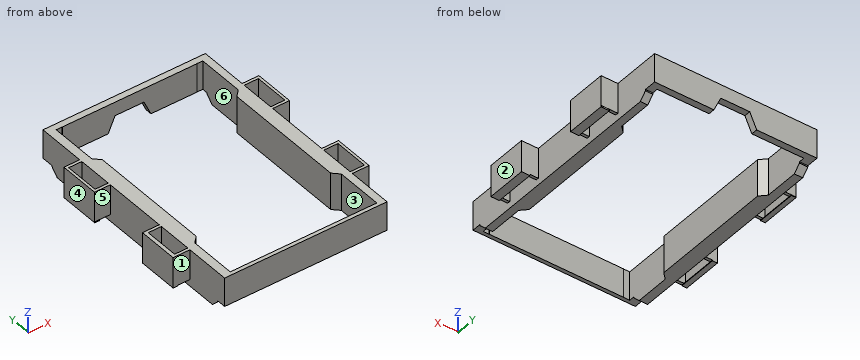
```python
from build123d import *

# Parameters (mm, degrees)
F0_W          = 60.96
F0_H          = 91.44
F0_W_2        = 50.8
F0_H_2        = 86.614
F1_DEPTH      = 28.448
F3_DEPTH      = 25.4
F4_W          = 66.649839282
F4_H          = 6.9823637605
F5_DEPTH      = 3.048
F6_W          = 64.9686481762
F6_H          = 4.777956934
F7_DEPTH      = 3.048
F9_DEPTH      = 2.286
F10_W         = 99.848318845
F10_H         = 48.2080141082
F11_DEPTH     = 50.8
F13_T1_DEPTH  = 15.8581495789
F13_T3_DEPTH  = 15.8581495789
F13_T8_DEPTH  = 41.5121495789
F13_T13_DEPTH = 41.5121495789
F13_T18_DEPTH = 41.5121495789
F13_T23_DEPTH = 41.5121495789
F14_W         = 15.24
F14_H         = 23.368
F15_DEPTH     = 6.35
F16_W         = 5.3607832682
F16_H         = 13.1506472826
F17_DEPTH     = 25.909
F19_DEPTH     = 0.254
F20_DEPTH     = 0.254
F21_DEPTH     = 1.016
F22_W         = 3.175
F22_H         = 15.24
F22_H_2       = 15.425526537
F23_DEPTH     = 0.508
F24_W         = 3.175
F24_H         = 15.24
F24_H_2       = 15.1729788631
F25_DEPTH     = 0.508
F26_W         = 1.4869117904
F26_H         = 15.24
F26_H_2       = 15.1544166729
F27_DEPTH     = 0.508
F28_W         = 1.5113
F28_H         = 15.24
F28_W_2       = 1.492887156
F28_H_2       = 15.3870563954
F29_DEPTH     = 0.254
F30_DEPTH     = 0.381
F31_DEPTH     = 0.254
F32_W         = 105.9566885233
F32_H         = 116.2753328681
F33_DEPTH     = 14.5


# Not quite as in the source:
# - a fillet or chamfer that OpenCascade refuses, or shapes differently, is made with other operations: its cross-section is extruded or revolved along the edge and cut away or added
# - a feature names something its author has since deleted; it is built from what else it names


with BuildPart() as f1:
    # F0 (on Top) → F1 (new body)
    with BuildSketch(Plane.XY):
        Rectangle(F0_W, F0_H)
        Rectangle(F0_W_2, F0_H_2, mode=Mode.SUBTRACT)
    extrude(amount=F1_DEPTH)

    # F2 (on face) → F3 (cut)
    with BuildSketch(Plane(origin=(0, 45.72, 0), x_dir=(-1, 0, 0), z_dir=(0, 1, 0))):
        Polygon((-9.4803553075, 0), (0, 0), (9.4803553075, 0), (5.461, 8.763), (-5.461, 8.763), align=None)
        Polygon((-9.4803553075, 28.448), (-5.461, 19.685), (5.461, 19.685), (9.4803553075, 28.448), (0, 28.448), align=None)
    extrude(amount=-F3_DEPTH, mode=Mode.SUBTRACT)

    # F4 (on Top) → F5 (cut)
    with BuildSketch(Plane.XY):
        with Locations((-0.1057945192, 44.6448102593)):
            Rectangle(F4_W, F4_H)
        with Locations((-0.1057945192, -44.6448102593)):
            Rectangle(F4_W, F4_H)
    extrude(amount=F5_DEPTH, mode=Mode.SUBTRACT)

    # F6 (on face) → F7 (cut)
    with BuildSketch(Plane.XY.offset(28.448)):
        with Locations((-2.0043240881, 43.331021533)):
            Rectangle(F6_W, F6_H)
        with Locations((-2.0043240881, -43.331021533)):
            Rectangle(F6_W, F6_H)
    extrude(amount=-F7_DEPTH, mode=Mode.SUBTRACT)

    # F8 (on face) → F9 (cut)
    with BuildSketch(Plane(origin=(25.4, 0, 0), x_dir=(0, -1, 0), z_dir=(-1, 0, 0))):
        Polygon((-43.0863499641, 0), (-41.1536283791, 0), (-25.9136283791, 0), (-25.9136283791, 30.48), (-41.1536283791, 30.48), (-43.0863499641, 30.48), align=None)
        Polygon((25.9136283791, 30.48), (25.9136283791, 0), (41.1536283791, 0), (43.0863499641, 0), (43.0863499641, 30.48), (41.1536283791, 30.48), align=None)
    extrude(amount=-F9_DEPTH, mode=Mode.SUBTRACT)

    # F10 (on Right) → F11 (cut)
    with BuildSketch(Plane.YZ):
        with Locations((1.7518345267, 13.4315635078)):
            Rectangle(F10_W, F10_H)
    extrude(amount=-F11_DEPTH, mode=Mode.SUBTRACT)

    # F12: F1 across plane


with BuildPart() as f1_1:
    add(f1.part)
    add(f1.part.mirror(Plane.YZ))

    # F13: chamfer of 2.54 on 12 edges, made by hand

    # F13_s2 → F13_t1 (cut)
    with BuildSketch(Plane.YZ.offset(-37.0120747894)):
        Polygon((38.402043066, 28.448), (40.942043066, 25.908), (40.942043066, 28.448), align=None)
        Polygon((38.6136283791, 0), (41.1536283791, 2.54), (41.1536283791, 0), align=None)
        Polygon((-40.942043066, 25.908), (-38.402043066, 28.448), (-40.942043066, 28.448), align=None)
        Polygon((-38.6136283791, 0), (-41.1536283791, 2.54), (-41.1536283791, 0), align=None)
    extrude(amount=F13_T1_DEPTH, mode=Mode.SUBTRACT)

    # F13_s4 → F13_t3 (cut)
    with BuildSketch(Plane.YZ.offset(21.1539252106)):
        Polygon((38.402043066, 28.448), (40.942043066, 25.908), (40.942043066, 28.448), align=None)
        Polygon((-40.942043066, 25.908), (-38.402043066, 28.448), (-40.942043066, 28.448), align=None)
        Polygon((-38.6136283791, 0), (-41.1536283791, 2.54), (-41.1536283791, 0), align=None)
        Polygon((38.6136283791, 0), (41.1536283791, 2.54), (41.1536283791, 0), align=None)
    extrude(amount=F13_T3_DEPTH, mode=Mode.SUBTRACT)


with BuildPart() as f13_tool6:
    # F13_s7 → F13_t8 (new body)
    with BuildSketch(Plane.XY.offset(-6.5320747894)):
        Polygon((25.4, 23.3736283791), (27.94, 25.9136283791), (25.4, 25.9136283791), align=None)
    extrude(amount=F13_T8_DEPTH)

    split(bisect_by=Plane.YZ.offset(27.686), keep=Keep.BOTTOM)


with BuildPart() as f1_2:
    add(f1_1.part)

    # F13_t5: cut F13_tool6
    add(f13_tool6.part, mode=Mode.SUBTRACT)


with BuildPart() as f13_tool11:
    # F13_s12 → F13_t13 (new body)
    with BuildSketch(Plane.XY.offset(34.9800747894)):
        Polygon((25.4, -23.3736283791), (27.94, -25.9136283791), (25.4, -25.9136283791), align=None)
    extrude(amount=-F13_T13_DEPTH)

    split(bisect_by=Plane.YZ.offset(27.686), keep=Keep.BOTTOM)


with BuildPart() as f1_3:
    add(f1_2.part)

    # F13_t10: cut F13_tool11
    add(f13_tool11.part, mode=Mode.SUBTRACT)


with BuildPart() as f13_tool16:
    # F13_s17 → F13_t18 (new body)
    with BuildSketch(Plane.XY.offset(-6.5320747894)):
        Polygon((-27.94, 25.9136283791), (-25.4, 23.3736283791), (-25.4, 25.9136283791), align=None)
    extrude(amount=F13_T18_DEPTH)

    split(bisect_by=Plane.YZ.offset(-27.686), keep=Keep.TOP)


with BuildPart() as f1_4:
    add(f1_3.part)

    # F13_t15: cut F13_tool16
    add(f13_tool16.part, mode=Mode.SUBTRACT)


with BuildPart() as f13_tool21:
    # F13_s22 → F13_t23 (new body)
    with BuildSketch(Plane.XY.offset(34.9800747894)):
        Polygon((-25.4, -23.3736283791), (-27.94, -25.9136283791), (-25.4, -25.9136283791), align=None)
    extrude(amount=-F13_T23_DEPTH)

    split(bisect_by=Plane.YZ.offset(-27.686), keep=Keep.TOP)


with BuildPart() as f1_5:
    add(f1_4.part)

    # F13_t20: cut F13_tool21
    add(f13_tool21.part, mode=Mode.SUBTRACT)

    # F14 (on face) → F15 (join)
    with BuildSketch(Plane.YZ.offset(30.48)):
        with Locations((-19.812, 14.224)):
            Rectangle(F14_W, F14_H)
        with Locations((19.812, 14.224)):
            Rectangle(F14_W, F14_H)
    extrude(amount=F15_DEPTH)

    # F16 (on face) → F17 (cut, through all)
    with BuildSketch(Plane.XY.offset(25.908)):
        with Locations((33.1603916341, -19.8066011071)):
            Rectangle(F16_W, F16_H)
        with Locations((33.1603916341, 19.8066011071)):
            Rectangle(F16_W, F16_H)
    extrude(amount=-F17_DEPTH, mode=Mode.SUBTRACT)

    # F18: F1 across plane


with BuildPart() as f1_6:
    add(f1_5.part)
    add(f1_5.part.mirror(Plane.YZ))

    # F19 (cut): faces of the model
    f19_faces = [f1_6.faces().sort_by_distance(p)[0] for p in [
        (26.543, -43.0863499641, 14.224),
        (-26.543, -43.0863499641, 14.224),
    ]]
    extrude(f19_faces, amount=-F19_DEPTH, mode=Mode.SUBTRACT)

    # F20 (cut): faces of the model
    f20_faces = [f1_6.faces().sort_by_distance(p)[0] for p in [
        (26.543, 43.0863499641, 14.224),
        (-26.543, 43.0863499641, 14.224),
    ]]
    extrude(f20_faces, amount=-F20_DEPTH, mode=Mode.SUBTRACT)

    # F21 (cut): a face of the model
    f21_faces = [f1_6.faces().sort_by_distance(p)[0] for p in [
        (0, -45.72, 14.224),
    ]]
    extrude(f21_faces, amount=-F21_DEPTH, mode=Mode.SUBTRACT)

    # F22 (on face) → F23 (join)
    with BuildSketch(Plane.XY.offset(25.908)):
        with Locations((-35.2425, 19.812)):
            Rectangle(F22_W, F22_H)
        with Locations((-35.2425, -19.7230628692)):
            Rectangle(F22_W, F22_H_2)
    extrude(amount=F23_DEPTH)

    # F24 (on face) → F25 (join)
    with BuildSketch(Plane(origin=(0, 0, 2.54), x_dir=(1, 0, 0), z_dir=(0, 0, -1))):
        with Locations((35.2425, 19.812)):
            Rectangle(F24_W, F24_H)
        with Locations((35.2425, -19.7903430089)):
            Rectangle(F24_W, F24_H_2)
    extrude(amount=F25_DEPTH)

    # F26 (on face) → F27 (join)
    with BuildSketch(Plane.XY.offset(25.908)):
        with Locations((36.0865441048, -19.812)):
            Rectangle(F26_W, F26_H)
        with Locations((36.0865441048, 19.7994005866)):
            Rectangle(F26_W, F26_H_2)
    extrude(amount=F27_DEPTH)

    # F28 (on face) → F29 (join)
    with BuildSketch(Plane(origin=(0, 0, 2.54), x_dir=(1, 0, 0), z_dir=(0, 0, -1))):
        with Locations((-36.07435, 19.812)):
            Rectangle(F28_W, F28_H)
        with Locations((-36.083556422, -19.7531366721)):
            Rectangle(F28_W_2, F28_H_2)
    extrude(amount=F29_DEPTH)

    # F30 (add): faces of the model
    f30_faces = [f1_6.faces().sort_by_distance(p)[0] for p in [
        (-30.48, 0.4258489378, 14.2172059936),
        (-35.3187, -19.812, 2.413),
        (-35.8407832682, -19.8066011071, 14.224),
        (-36.83, -19.8101053315, 14.3540262363),
    ]]
    extrude(f30_faces, amount=F30_DEPTH, dir=(-1, 0, 0))

    # F31 (add): a face of the model
    f31_faces = [f1_6.faces().sort_by_distance(p)[0] for p in [
        (-35.337112844, 19.7531366721, 2.413),
    ]]
    extrude(f31_faces, amount=F31_DEPTH)

    # F32 (on face) → F33 (cut)
    with BuildSketch(Plane.XY.offset(28.448)):
        with Locations((11.0789313912, -7.9427920282)):
            Rectangle(F32_W, F32_H)
    extrude(amount=-F33_DEPTH, mode=Mode.SUBTRACT)


solid = f1_6.part
```
Geometry: final body of the model. Coordinates: model frame, mm. Face numbers are marked on the shaded views. A direction names the side the tool comes from. Coordinates: 2 decimals unless noted, no trailing zeros. Order: outer loops, then holes, each group sorted by start corner. A loop starts at its lowest first (then second) coordinate and runs counter-clockwise, first axis right, second up.
Item 1: Section query D-D (z = 10.5). State how many separate pieces and enclosed holes the cut face has, then the cut area to 3 significant figures.
Answer:
separate pieces: 1
enclosed holes: 5
area: 1,080 mm2
Item 2: Draft query along Y for the marked faces 1, 2 and 3. Return one class per face: released by +Y, released by -Y, zero draft, split by the parting line, or undercut.
Answer:
face 1: released by -Y
face 2: zero draft
face 3: undercut
Item 3: Material intervals for line 1 along X through (y, z) = (-26, 3.5); line 2 along X through (y, z) = (-22.5, 7.5); line 3 along Y through (x, z) = (-31.5, 6), sorted ascending.
Answer:
line 1: x = -37.21 to -35.84, -30.86 to -27.69, 27.69 to 30.48, 35.84 to 36.83
line 2: x = -37.21 to -35.84, -30.86 to -25.4, 25.4 to 30.48, 35.84 to 36.83
line 3: y = -27.43 to -26.38, -13.23 to -12.19, 12.19 to 13.23, 26.38 to 27.43
Item 4: Access query for the marked faces 4, 5 and 6. Directions: +Z, -Z, +X, -X, +Y, -Y. A direction counts if a zero-diameter tool reaches every point of the face in a straight line with its end or side. Return the directions, or none.
Answer:
face 4: +Z, -Z, -X, +Y
face 5: +Z, -X
face 6: +Z, -Z
Item 5: Section query B-B (x = 2.5). Output: boundary loops of the cut face in (y, z), then the cut area to 3 significant figures.
Answer:
outline: (-44.7, 3.05) - (-43.31, 3.05) - (-43.31, 13.95) - (-44.7, 13.95) - close; (43.31, 8.76) - (45.72, 8.76) - (45.72, 13.95) - (43.31, 13.95) - close
area: 27.7 mm2
Item 6: Section query C-C (y = -17.5). Output: boundary loops of the cut face in (x, z) (3 decimals).
Answer:
outline: (-37.211, 2.286) - (-35.319, 2.286) - (-35.319, 2.54) - (-35.841, 2.54) - (-35.841, 13.948) - (-37.211, 13.948) - close; (-30.861, 0) - (-25.4, 0) - (-25.4, 13.948) - (-30.861, 13.948) - close; (25.4, 0) - (30.48, 0) - (30.48, 13.948) - (25.4, 13.948) - close; (33.655, 2.032) - (36.83, 2.032) - (36.83, 13.948) - (35.841, 13.948) - (35.841, 2.54) - (33.655, 2.54) - close
Item 7: Contact query for flat-ended pins moving along their axis: P1, Ø2.5, axis at x = -33.5, z = 10.5, coming from the +Y side; P2, Ø3, axis at x = 12.5, y = -42.5, coming from the -Z side; P3, Ø4, axis at x = -34, z = 9, coming from the -Y side; P4, Ø5, axis at x = 28.5, y = 28, coming from the -Z side. Output: stop coordinate, or through.
Answer:
P1: stops at y = 27.43
P2: stops at z = 3.05
P3: stops at y = -27.43
P4: stops at z = 0
Item 8: Section query A-A (y = 31.5). Output: boundary loops of the cut face in (x, z).
Answer:
outline: (-30.86, 0) - (-27.69, 0) - (-27.69, 13.95) - (-30.86, 13.95) - close; (27.69, 0) - (30.48, 0) - (30.48, 13.95) - (27.69, 13.95) - close
